from build123d import *

# Parameters (mm, degrees)
F2_DEPTH = 158.75
F3_R     = 3.96875
F4_DEPTH = 19.051


with BuildPart() as f2:
    # F1 (on offset) → F2 (new body)
    with BuildSketch(Plane.YZ.offset(78.58125)):
        Polygon((-7.9375, 79.375), (-9.525, 79.375), (-9.525, -79.375), (-7.9375, -79.375), (-7.9375, -68.2625), (7.9375, -68.2625), (7.9375, -79.375), (9.525, -79.375), (9.525, 79.375), (7.9375, 79.375), (7.9375, 68.2625), (-7.9375, 68.2625), align=None)
    extrude(amount=-F2_DEPTH)

    # F3 (on face) → F4 (cut, through all)
    with BuildSketch(Plane(origin=(0, 9.525, 0), x_dir=(-1, 0, 0), z_dir=(0, 1, 0))):
        with Locations((66.675, 66.675)):
            Circle(F3_R)
        with Locations((-66.675, 66.675)):
            Circle(F3_R)
        with Locations((-66.675, -66.675)):
            Circle(F3_R)
        with Locations((66.675, -66.675)):
            Circle(F3_R)
    extrude(amount=-F4_DEPTH, mode=Mode.SUBTRACT)


solid = f2.part
Can you work these out from the model? Positions are in its coordinate system, mm. A direction names the side the tool comes from. Give positions to 0.01 mm unless a question says otherwise; leave off trailing zeros. Order: outer loops, then holes, each group sorted by start corner. A loop starts at its lowest first (then second) coordinate and runs counter-clockwise, first axis right, second up. Notation, with made-up numbers: M -27.75,68.25 L -23.75,68.25 A30 ccw -23.75,91.25 Z; hole C 53,85 d11. An arc over 180 degrees is marked long. One line per item, written item: value.
Item 1: If we mould it in two halves opening along X, with no side actions, what happens to faces 4 (the face through (78.581, 0, 1)), 5 (the face through (67.19, 0.13, -62.74)), 6 (the face through (75, 0, 68.262))? For each: pulls with the +X half, pulls with the -X half, needs draft (parallel to the pull), parting line crosses it, or undercut.
Verdict:
face 4: pulls with the +X half
face 5: undercut
face 6: needs draft
Item 2: For pin 1 (8 mm diameter, centred on x = 2.5, y = 3.5, fed in from -Z); pin 2 (10.5 mm diameter, centred on x = -66.675, z = -66.675, fed in from -Y) (3 decimals); pin 3 (9 mm diameter, centred on x = 76.5, y = 0.5, fed in from +Z); pin 4 (5 mm diameter, centred on x = -66.675, z = 66.675, fed in from -Y), each with a flat end and sliding along its axis, tell me the tip position at first contact or that it passes through.
Verdict:
pin 1: z = -68.26
pin 2: y = -9.525
pin 3: z = 68.26
pin 4: through
Item 3: For faces 1 (the face through (0, -7.938, -74)), 2 (the face through (-75, 0, 68.262)), 3 (the face through (0, -9.525, 1)), which set-ups out of +Z, -Z, +X, -X, +Y, -Y let a thin tool reach every point of the face, with its end or its side?
Verdict:
face 1: -Z, +X, -X
face 2: +Z, +X, -X
face 3: +Z, -Z, +X, -X, -Y
Item 4: If we section it at C-C on x = 68.5: Write out the boundary of the cut face in (y, z) (1 decimal).
Verdict:
outline: M -9.5,-79.4 L -7.9,-79.4 L -7.9,-70.2 L -9.5,-70.2 Z; M -9.5,-63.2 L 9.5,-63.2 L 9.5,63.2 L -9.5,63.2 Z; M -9.5,70.2 L -7.9,70.2 L -7.9,79.4 L -9.5,79.4 Z; M 7.9,-79.4 L 9.5,-79.4 L 9.5,-70.2 L 7.9,-70.2 Z; M 7.9,70.2 L 9.5,70.2 L 9.5,79.4 L 7.9,79.4 Z
Item 5: If we section it at B-B on y = 2.75: Write out the boundary of the cut face in (x, z) (1 decimal), and give its area (3 significant figures).
Verdict:
outline: M -80.2,-68.3 L -70.3,-68.3 A4 cw long -63,-68.3 L 63,-68.3 A4 cw long 70.3,-68.3 L 78.6,-68.3 L 78.6,68.3 L 70.3,68.3 A4 cw long 63,68.3 L -63,68.3 A4 cw long -70.3,68.3 L -80.2,68.3 Z
area: 21,500 mm2
Item 6: If we section it at A-A on x = 43: Write out the boundary of the cut face in (y, z) (1 decimal), and give its area (3 significant figures).
Verdict:
outline: M -9.5,-79.4 L -7.9,-79.4 L -7.9,-68.3 L 7.9,-68.3 L 7.9,-79.4 L 9.5,-79.4 L 9.5,79.4 L 7.9,79.4 L 7.9,68.3 L -7.9,68.3 L -7.9,79.4 L -9.5,79.4 Z
area: 2,670 mm2
Item 7: Please list where these lines run through material, in increasing order: line 1 (Z direction, x = -44.5, y = 6.75); line 2 (Z direction, x = -65, y = -4).
Verdict:
line 1: -68.26 to 68.26
line 2: -63.08 to 63.08
Item 8: If we section it at D-D on x = -65: Write out the boundary of the cut face in (y, z) (1 decimal), and give its area (3 significant figures).
Verdict:
outline: M -9.5,-79.4 L -7.9,-79.4 L -7.9,-70.3 L -9.5,-70.3 Z; M -9.5,-63.1 L 9.5,-63.1 L 9.5,63.1 L -9.5,63.1 Z; M -9.5,70.3 L -7.9,70.3 L -7.9,79.4 L -9.5,79.4 Z; M 7.9,-79.4 L 9.5,-79.4 L 9.5,-70.3 L 7.9,-70.3 Z; M 7.9,70.3 L 9.5,70.3 L 9.5,79.4 L 7.9,79.4 Z
area: 2,460 mm2
